Work out the finished part from the listing and answer in its coordinate system (mm). A direction names the side the tool comes from. Coordinates: 2 decimals unless noted, no trailing zeros. Write each loop counter-clockwise with the first axis right and the second up, starting at its lowest first coordinate (ties: lowest second). Pieces come first, ordered by that corner, then holes. Notation, with made-up numbers: M 48,-32 L 98,-32 A22 ccw 98,-20 Z; hole C 34.5,64.5 d5. An arc over 180 degrees is marked long. Answer as CSV lines item,"result". Start each with the question number.
(1) For faces 4 (the flat face through (4, 74.5, 49)), 5 (the cylindrical face through (286.091, -6.457, 49.3)), 6 (the cylindrical face through (11.909, 6.457, 49.3)), determine the directions among +Z, -Z, +X, -X, +Y, -Y from which every point of the face is accessible in a straight line to the end or side of a thin tool.
(2) The mould has two halves that part along X. Classify faces 1 (the flat face through (0, 1, 49)), 2 (the flat face through (294, 74.5, 49)), 3 (the flat face through (8, 45, 49)): released by +X, released by -X, zero draft, split by the parting line, or undercut.
(3) A cutting plane is placed at B-B on z = 21. Give the vertices of the cut face in (x, y).
(4) Find the intervals of material crossed by L1, parallel to X at y = 67, z = 14; L2, parallel to Y at x = 173, z = 93; L3, parallel to X at y = -9, z = 94, in increasing order. Write a range as [from, to].
(5) A cutting plane is placed at A-A on y = 19. Give the vertices of the cut face in (x, z), then the cut area to 3 significant figures.
(6) A cutting plane is placed at C-C on x = 211.5. Give the vertices of the cut face in (y, z), then the cut area to 3 significant figures.
Autodesk Fusion 360 part; units mm, degrees
sketch "スケッチ1" plane through (0, 0, 0) normal (0, 0, 1) x (1, 0, 0)
  line L0 (0, 74.5) -> (0, -74.5)
  line L1 (298, -74.5) -> (298, 74.5)
  line L2 (290, -15.75) -> (290, -74.5)
  line L3 (8, -74.5) -> (8, -15.75)
  line L4 (0, -74.5) -> (8, -74.5)
  line L5 (290, -74.5) -> (298, -74.5)
  line L6 (277, 2.75) -> (21, 2.75)
  line L7 (21, -2.75) -> (277, -2.75)
  line L8 (8, 15.75) -> (8, 74.5)
  arc A0 (8, 15.75) -> (21, 2.75) centre (21, 15.75) ccw
  arc A1 (21, -2.75) -> (8, -15.75) centre (21, -15.75) ccw
  line L9 (8, 74.5) -> (0, 74.5)
  line L10 (290, 74.5) -> (290, 15.75)
  arc A2 (277, 2.75) -> (290, 15.75) centre (277, 15.75) ccw
  arc A3 (290, -15.75) -> (277, -2.75) centre (277, -15.75) ccw
  line L11 (298, 74.5) -> (290, 74.5)
extrude "押し出し1" add sketch "スケッチ1" along normal blind 100
Here are the results:
1,face 4,"+Z, -Z, +X, -X, +Y"
1,face 5,"+Z, -Z, -Y"
1,face 6,"+Z, -Z, +Y"
2,face 1,"released by -X"
2,face 2,"zero draft"
2,face 3,"undercut"
3,outline,"M 0,-74.5 L 8,-74.5 L 8,-15.75 A13 cw 21,-2.75 L 277,-2.75 A13 cw 290,-15.75 L 290,-74.5 L 298,-74.5 L 298,74.5 L 290,74.5 L 290,15.75 A13 cw 277,2.75 L 21,2.75 A13 cw 8,15.75 L 8,74.5 L 0,74.5 Z"
4,L1,"x = [0, 8], [290, 298]"
4,L2,"y = [-2.75, 2.75]"
4,L3,"x = [0, 9.89], [288.11, 298]"
5,outline,"M 0,0 L 8,0 L 8,100 L 0,100 Z; M 290,0 L 298,0 L 298,100 L 290,100 Z"
5,area,"1,600 mm^2"
6,outline,"M -2.75,0 L 2.75,0 L 2.75,100 L -2.75,100 Z"
6,area,"550 mm^2"
